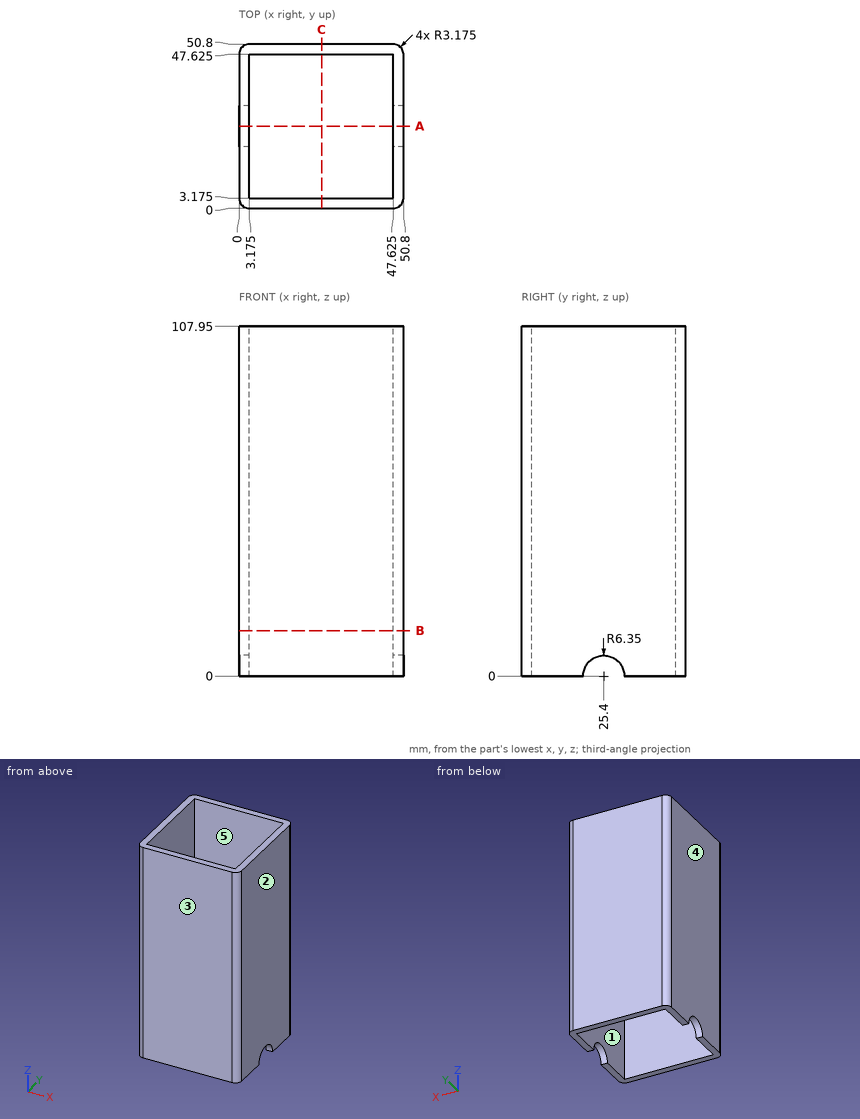
Drawing for the job (mm, zero at the part's lowest x, y, z). A direction names the side the tool comes from. Give positions to 0.01 mm unless a question says otherwise; leave off trailing zeros. Order: outer loops, then holes, each group sorted by start corner. A loop starts at its lowest first (then second) coordinate and runs counter-clockwise, first axis right, second up. Notation, with made-up numbers: (24.5, 23) - (42.5, 23) arc R16 ccw to (42.5, 44) - close; hole circle Ø8 at (-4.5, 77.5). An arc over 180 degrees is marked (long way). Use one line per item in the form item = value.
Item 1: Slice it at A-A on y = 25.4. Give the cut face in (x, z) (3 decimals), and give its area (3 significant figures).
Solution:
outline = (0, 6.35) - (3.175, 6.35) - (3.175, 107.95) - (0, 107.95) - close; (47.625, 6.35) - (50.8, 6.35) - (50.8, 107.95) - (47.625, 107.95) - close
area = 645 mm2
Item 2: Which spindle directions (+Z, -Z, +X, -X, +Y, -Y) get a long thin tool onto all of the face, cutting with end or side? Do the marked faces 1 and 2. Say none if no direction does.
Solution:
face_1 = +Z, -Z
face_2 = +Z, -Z, +X, +Y, -Y
Item 3: Probe probe 1 along X at (y, z) = (32, 91.5) (3 decimals); probe 2 along X at (y, z) = (3, 66.5). List the from-to ranges inside material, lowest first. Write a range as from..to.
Solution:
probe_1 = 0..3.175, 47.625..50.8
probe_2 = 0..50.8
Item 4: Slice it at C-C on x = 25.5. Give the cut face in (y, z) (3 decimals).
Solution:
outline = (0, 0) - (3.175, 0) - (3.175, 107.95) - (0, 107.95) - close; (47.625, 0) - (50.8, 0) - (50.8, 107.95) - (47.625, 107.95) - close
Item 5: Slice it at B-B on z = 14. Give the cut face in (x, y) (3 decimals), and give its area (3 significant figures).
Solution:
outline = (0, 3.175) arc R3.175 ccw to (3.175, 0) - (47.625, 0) arc R3.175 ccw to (50.8, 3.175) - (50.8, 47.625) arc R3.175 ccw to (47.625, 50.8) - (3.175, 50.8) arc R3.175 ccw to (0, 47.625) - close; hole (3.175, 3.175) - (47.625, 3.175) - (47.625, 47.625) - (3.175, 47.625) - close
area = 596 mm2
Item 6: Two-plate mould, pull along Y, no slides. Class the marked faces 3, 4 and 5: released by +Y, released by -Y, zero draft, split by the parting line, or undercut.
Solution:
face_3 = released by -Y
face_4 = zero draft
face_5 = undercut
